The model under review builds one solid part; all positions refer to its coordinate system, in mm. A direction names the side the tool comes from. Give positions to 0.01 mm unless a question says otherwise; leave off trailing zeros. Loops run counter-clockwise (first coordinate to the right, second up) from the corner with the lowest first, then second, coordinate; pieces in that order, holes last. Notation, with made-up numbers: M 83.25,23 L 99.25,23 A26 cw 99.25,38 Z; hole C 27.25,38.5 d2. An arc over 180 degrees is marked long. Write item = value, one per line. Start each with the question number.
1. We need section A-A on x = 13.5. Give the boundary of the cut face in (y, z), then the cut area to 3 significant figures.
2. Wall thickness on line 1 along X through (y, z) = (8.3, -27.5); line 2 along Y through (x, z) = (10.5, 30); line 3 along Z through (x, y) = (7.5, 1.95): over which ranges is each line inside the solid? List them lowest first. Write a range as from..to.
3. We need section C-C on z = 23.5. Give the boundary of the cut face in (x, y), then the cut area to 3 significant figures.
4. Draft analysis for pull direction Z (two halves, no side actions). For faces 1 (the face through (7.605, 4.503, -4.52)), 2 (the face through (7.4, 3, 30.5)), 3 (the face through (0, 5, 0)), state which applies: pulls with the +Z half, pulls with the -Z half, needs draft (parallel to the pull), parting line crosses it, or undercut.
5. For faces 4 (the face through (7, 6, 22)), 5 (the face through (7, 0, 21)), 6 (the face through (7, 5, -21)), list the 3-axis set-ups (+Z, -Z, +X, -X, +Y, -Y) from which the entire face can be reached by the end or side of a thin tool; tool diameter is ignored.
6. For pin 1 (6 mm diameter, centred on x = 2.5, z = 25, fed in from +Y); pin 2 (2 mm diameter, centred on y = 4.5, z = -25.5, fed in from +X); pin 3 (1.5 mm diameter, centred on x = 2.5, z = -27, fed in from -Y), all flat-tipped, find the tip position at first contact; note any pin that passes through.
Autodesk Inventor part; units mm, degrees
ref_plane "YZ Plane" through (0, 0, 0) normal (1, 0, 0) x (0, 1, 0)
ref_plane "XZ Plane" through (0, 0, 0) normal (0, 1, 0) x (-1, 0, 0)
ref_plane "XY Plane" through (0, 0, 0) normal (0, 0, 1) x (1, 0, 0)
sketch "Sketch1" plane through (0, 0, 0) normal (1, 0, 0) x (0, 1, 0)
  line L0 (0, 4.3301) -> (0, 35)
  line L1 (0, 35) -> (6, 35)
  line L2 (6, 35) -> (6, 4.3301)
  line L3 (5, -4.3301) -> (5, -35)
  line L4 (5, -35) -> (11, -35)
  line L5 (11, -35) -> (11, -4.3301)
  line L6 (0, 4.3301) -> (5, -4.3301)
  line L7 (2.5, 0) -> (6, 0) construction
  line L8 (6, 4.3301) -> (11, -4.3301)
  point P0 (0, 0)
  dimension "d1" = 6
  dimension "d11" = 6
extrude "Extrusão1" add sketch "Sketch1" along normal blind 15
fillet "Arredondamento1" radius 15 4 edges at (7.5, 11, -4.3301) (7.5, 6, 4.3301) (7.5, 0, 4.3301) (7.5, 5, -4.3301)
fillet "Arredondamento2" radius 7.5 4 edges at (15, 3, 35) (0, 3, 35) (15, 8, -35) (0, 8, -35)
sketch "Esboço2" plane through (0, 0, 8.3494) normal (0, -1, 0) x (1, 0, 0)
  line L0 (0, -9.1987) -> (15, -9.1987)
  arc A0 (15, 19.1506) -> (0, 19.1506) centre (7.5, 19.1506) ccw
  arc A1 (0, -35.8494) -> (15, -35.8494) centre (7.5, -35.8494) ccw
  circle A2 centre (7.5, 19.1506) radius 3
  circle A3 centre (7.5, -35.8494) radius 3
  point P0 (0, -8.3494)
  dimension "d29" = 6
  dimension "d31" = 6
hole "Furo1" at (7.5, 0, 27.5) at (7.5, 0, -27.5) direction (0, 1, 0) diameter 6 end through all
properties part number "jumelo"
Final values:
q1.outline = M 0,8.35 A15 ccw 2.01,0.85 L 2.99,-0.85 A15 cw 5,-8.35 L 5,-32 L 11,-32 L 11,-8.35 A15 ccw 8.99,-0.85 L 8.01,0.85 A15 cw 6,8.35 L 6,32 L 0,32 Z
q1.area = 384 mm²
q2.line_1 = 0..4.5, 10.5..15
q2.line_2 = 0..6
q2.line_3 = 0.95..24.5, 30.5..35
q3.outline = M 0,0 L 15,0 L 15,6 L 0,6 Z
q3.area = 90.0 mm²
q4.face_1 = pulls with the -Z half
q4.face_2 = undercut
q4.face_3 = needs draft
q5.face_4 = +Z, +X, -X, +Y
q5.face_5 = +Z, -Z, +X, -X, -Y
q5.face_6 = -Z, +X, -X, -Y
q6.pin_1 = 6
q6.pin_2 = 15
q6.pin_3 = 5
